Geometry: see drawing. Coordinates: mm, zero at the bounding-box minimum. A direction names the side the tool comes from. Give positions to 0.01 mm unless a question says otherwise; leave off trailing zeros. Loops run counter-clockwise (first coordinate to the right, second up) from the corner with the lowest first, then second, coordinate; pieces in that order, holes last. Notation, with made-up numbers: (40.5, -5) -> (72.5, -5) arc R18 ccw to (72.5, 24) -> close; hole circle Ø11 at (21.25, -25). An arc over 180 degrees is marked (long way). Use CSV: the item, a comma, the result in double quotes.
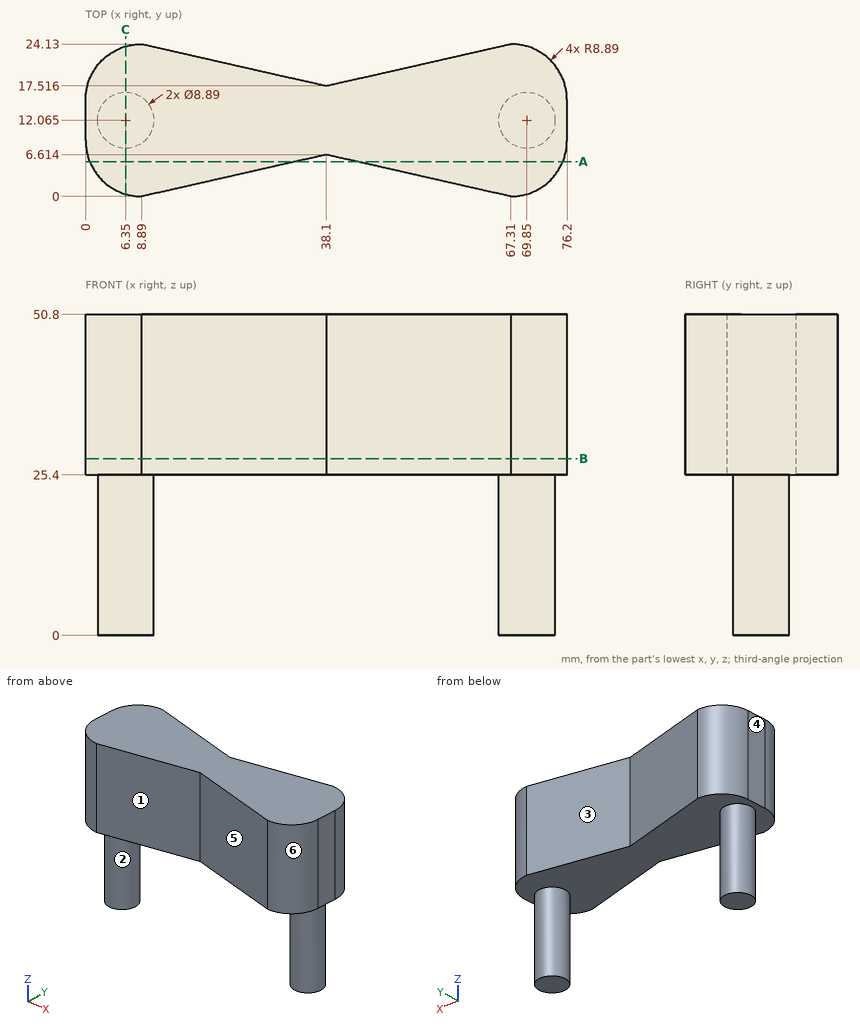
1) Section query A-A (y = 5.5). Return loops of the section in (x, z).
From the geometry:
outline,"(0.67, 25.4) -> (33.18, 25.4) -> (33.18, 50.8) -> (0.67, 50.8) -> close; (43.02, 25.4) -> (75.53, 25.4) -> (75.53, 50.8) -> (43.02, 50.8) -> close"
2) Section query C-C (x = 6.35). Return loops of the section in (y, z), then the cut area to 3 significant figures.
From the geometry:
outline,"(0.37, 25.4) -> (7.62, 25.4) -> (7.62, 0) -> (16.51, 0) -> (16.51, 25.4) -> (23.76, 25.4) -> (23.76, 50.8) -> (0.37, 50.8) -> close"
area,"820 mm^2"
3) Contact query for flat-ended pins moving along their axis: pin 1 (4 mm diameter, centred on y = 6, z = 19.5, fed in from -X); pin 2 (3 mm diameter, centred on y = 7, z = 21.5, fed in from -X) (1 decimal); pin 3 (10 mm diameter, centred on x = 26, y = 9, fed in from -Z). Output: stop coordinate, or through.
From the geometry:
pin 1,"stops at x = 4.55"
pin 2,"stops at x = 3.7"
pin 3,"stops at z = 25.4"
4) Section query B-B (z = 28). Return loops of the section in (x, y), then the cut area to 3 significant figures.
From the geometry:
outline,"(0, 8.89) arc R8.89 ccw to (8.89, 0) -> (38.1, 6.61) -> (67.31, 0) arc R8.89 ccw to (76.2, 8.89) -> (76.2, 15.24) arc R8.89 ccw to (67.31, 24.13) -> (38.1, 17.52) -> (8.89, 24.13) arc R8.89 ccw to (0, 15.24) -> close"
area,"1,380 mm^2"
5) Ray query, line 1 (Z direction, x = 12, y = 12.25); line 2 (X direction, y = 8.75, z = 9); line 3 (X direction, y = 13.75, z = 5). Return the intervals inside material, ascending.
From the geometry:
line 1,"z = 25.4 to 50.8"
line 2,"x = 3.39 to 9.31, 66.89 to 72.81"
line 3,"x = 2.24 to 10.46, 65.74 to 73.96"
6) Reachability of the marked faces 1, 2 and 3 from +Z, -Z, +X, -X, +Y, -Y: full face, straight path, thin tool, end or side. Return the list, or none.
From the geometry:
face 1,"+Z, -Z, -Y"
face 2,"-Z"
face 3,"+Z, -Z, +Y"
7) Mould query, pull axis X, two halves, no side actions, for the marked faces 4, 5 and 6. Classes: pulls with the +X half, pulls with the -X half, needs draft (parallel to the pull), parting line crosses it, or undercut.
From the geometry:
face 4,"pulls with the -X half"
face 5,"undercut"
face 6,"pulls with the +X half"
